from build123d import *

# Parameters (mm, degrees)
PAD_DEPTH       = 40
SKETCH001_R     = 11
POCKET_DEPTH    = 5
SKETCH002_R     = 1.6
POCKET001_DEPTH = 40.001
FILLET_R        = 2
POCKET002_DEPTH = 5
FILLET001_R     = 2


with BuildPart() as part:
    # Sketch → Pad (new body)
    with BuildSketch(Plane.YZ):
        Polygon((5, 5), (5, 58), (0, 58), (0, 0), (40, 0), (40, 5), align=None)
    extrude(amount=-PAD_DEPTH)

    # Sketch001 (on Face3 of Pad) → Pocket (cut)
    with BuildSketch(Plane(origin=(0, 0, 0), x_dir=(0, 0, -1), z_dir=(0, -1, 0))):
        with Locations((-38, -20)):
            Circle(SKETCH001_R)
    extrude(amount=-POCKET_DEPTH, mode=Mode.SUBTRACT)

    # Sketch002 (on Face8 of Pocket) → Pocket001 (cut, through all)
    with BuildSketch(Plane(origin=(0, 0, 0), x_dir=(0, 0, -1), z_dir=(0, -1, 0))):
        with Locations((-53, -20)):
            Circle(SKETCH002_R)
        with Locations((-30.5, -32.99)):
            Circle(SKETCH002_R)
        with Locations((-30.5, -7.01)):
            Circle(SKETCH002_R)
    extrude(amount=-POCKET001_DEPTH, mode=Mode.SUBTRACT)

    # Fillet
    fillet_edges = [part.edges().sort_by_distance(p)[0] for p in [
        (0, 2.5, 58),
        (-40, 2.5, 58),
    ]]
    fillet(fillet_edges, radius=FILLET_R)

    # Sketch003 (on Face4 of Fillet) → Pocket002 (cut)
    with BuildSketch(Plane(origin=(0, 0, 5), x_dir=(0, -1, 0), z_dir=(0, 0, 1))):
        with BuildLine():
            ThreePointArc((-32, -7.4), (-34.6, -10), (-32, -12.6))
            Line((-32, -12.6), (-22, -12.6))
            ThreePointArc((-22, -12.6), (-19.4, -10), (-22, -7.4))
            Line((-22, -7.4), (-32, -7.4))
        make_face()
        with BuildLine():
            ThreePointArc((-32, -27.4), (-34.6, -30), (-32, -32.6))
            Line((-32, -32.6), (-22, -32.6))
            ThreePointArc((-22, -32.6), (-19.4, -30), (-22, -27.4))
            Line((-22, -27.4), (-32, -27.4))
        make_face()
    extrude(amount=-POCKET002_DEPTH, mode=Mode.SUBTRACT)

    # Fillet001
    fillet001_edges = [part.edges().sort_by_distance(p)[0] for p in [
        (0, 40, 2.5),
        (-40, 40, 2.5),
    ]]
    fillet(fillet001_edges, radius=FILLET001_R)


solid = part.part
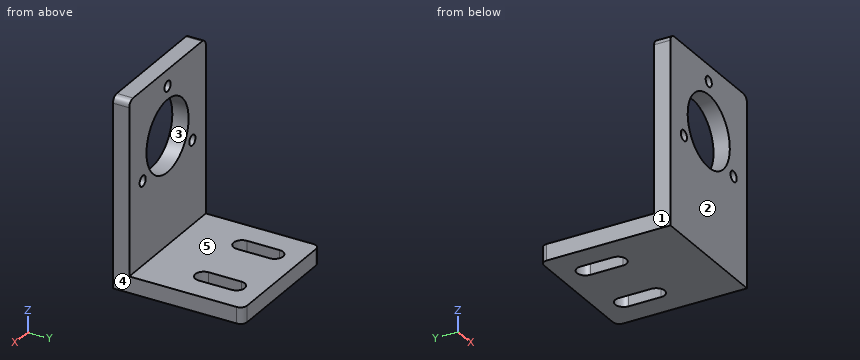
Build history of the part. All positions in model axes, mm. Face numbers are marked on the shaded views. A direction names the side the tool comes from. Coordinates: 2 decimals unless noted, no trailing zeros. Order: outer loops, then holes, each group sorted by start corner. A loop starts at its lowest first (then second) coordinate and runs counter-clockwise, first axis right, second up. Notation, with made-up numbers: M 26.25,22 L 81.25,22 A37 cw 81.25,58 Z; hole C 55.25,65 d1. An arc over 180 degrees is marked long. One line per question, with ' | ' between items. Start each with the question number.
Q1. Saw through at D-D (z = 30.5). List the corners of the cut face in (x, y), then the cut area to 3 significant figures.
Q2. Saw through at A-A (y = 27). List the corners of the cut face in (x, z).
Q3. Saw through at C-C (x = -20). List the corners of the cut face in (y, z), then the cut area to 3 significant figures.
Q4. Two-plate mould, pull along X, no slides. Class the marked faces 1, 2 and 3: +X half, -X half, draft (parallel to the pull), parting line (faces both ways), or undercut.
Q5. 3-axis set-ups, long thin cutter, end or side, ignore diameter. For the marked faces 4 and 5: which of +Z, -Z, +X, -X, +Y, -Y reach the whole face in a straight line?
Q6. Saw through at B-B (z = 53). List the corners of the cut face in (x, y).
Q7. Probe L1, parallel to X at y = 2.95, z = 30.5; L2, parallel to Y at x = -18, z = 17.5. List the from-to ranges inside material, lowest first. Write a range as from..to.
Q8. Flat gauge pins, fed straight in: pin 1 Ø1.5 at (x, z) = (-18, 8.5) entering from +Y; pin 2 Ø2 at (y, z) = (7.5, 9.5) entering from -X. Where does each tip first touch, or does it go through?
Check values:
1) outline: M -40,0 L -34.59,0 L -34.59,5 L -40,5 Z; M -31.39,0 L -28.05,0 L -28.05,5 L -31.39,5 Z; M -11.95,0 L -8.61,0 L -8.61,5 L -11.95,5 Z; M -5.41,0 L 0,0 L 0,5 L -5.41,5 Z | area: 87.5 mm2
2) outline: M -40,0 L -32.6,0 L -32.6,5 L -40,5 Z; M -27.4,0 L -12.6,0 L -12.6,5 L -27.4,5 Z; M -7.4,0 L 0,0 L 0,5 L -7.4,5 Z
3) outline: M 0,0 L 40,0 L 40,5 L 5,5 L 5,27 L 0,27 Z; M 0,49 L 5,49 L 5,51.4 L 0,51.4 Z; M 0,54.6 L 5,54.6 L 5,58 L 0,58 Z | area: 339 mm2
4) face 1: -X half | face 2: draft | face 3: undercut
5) face 4: +Z, -Z, +X, +Y, -Y | face 5: +Z, +X, -X, +Y
6) outline: M -40,0 L -21.6,0 L -21.6,5 L -40,5 Z; M -18.4,0 L 0,0 L 0,5 L -18.4,5 Z
7) L1: x = -40..-34.59, -31.39..-28.05, -11.95..-8.61, -5.41..0 | L2: y = 0..5
8) pin 1: stops at y = 5 | pin 2: passes through
